```python
from build123d import *

# Parameters (mm, degrees)
SKETCH1_W           = 4.5
SKETCH1_H           = 76
SKETCH2_W           = 19
SKETCH2_H           = 19
BOSS_EXTRUDE1_DEPTH = 6
CHAMFER2_SIZE       = 1
CHAMFER2_SIZE2      = 1.732050808


with BuildPart() as part:
    # Sketch1 → Revolve1 (revolve)
    with BuildSketch(Plane.XY, mode=Mode.PRIVATE) as revolve1_sk:
        with Locations((2.25, 38)):
            Rectangle(SKETCH1_W, SKETCH1_H)
    revolve(revolve1_sk.sketch.rotate(Axis((0, 0, 0), (0, 1, 0)), 90), axis=Axis((0, 0, 0), (0, 1, 0)))  # turned: the seam where the file's is

    # Sketch2 → Boss-Extrude1 (add)
    with BuildSketch(Plane(origin=(0, 0, 0), x_dir=(1, 0, 0), z_dir=(0, 1, 0))):
        Rectangle(SKETCH2_W, SKETCH2_H)
    extrude(amount=-BOSS_EXTRUDE1_DEPTH)

    # Chamfer2
    chamfer2_edges = [part.edges().sort_by_distance(p)[0] for p in [
        (0, 76, 4.5),
    ]]
    chamfer2_side = [part.faces().sort_by_distance(p)[0] for p in [
        (0, 76, 0),
    ]]
    chamfer(chamfer2_edges, length=CHAMFER2_SIZE, length2=CHAMFER2_SIZE2, reference=chamfer2_side[0])


solid = part.part
```
Input: part model. Units: mm. Frame: model coordinates. A direction names the side the tool comes from. Coordinates: 2 decimals unless noted, no trailing zeros. Write each loop counter-clockwise with the first axis right and the second up, starting at its lowest first coordinate (ties: lowest second). Pieces come first, ordered by that corner, then holes. Notation, with made-up numbers: (15.25, 89) - (54.25, 89) arc R20 ccw to (54.25, 105) - close; hole circle Ø1 at (56, -24.5). An arc over 180 degrees is marked (long way). Put each result on its own line as item: value. Start each with the question number.
1) Contact query for flat-ended pins moving along their axis: pin 1 (10 mm diameter, centred on y = 9, z = -2, fed in from -X); pin 2 (3 mm diameter, centred on x = 0.5, y = 53.5, fed in from +Z); pin 3 (8 mm diameter, centred on x = -3, y = 51.5, fed in from -Z). Output: stop coordinate, or through.
2) Cut plane B-B (z = 7.75). Return the cut outline in (x, y).
3) Cut plane A-A (x = 0). Return the cut outline in (y, z).
4) Cut plane D-D (x = -7.5). Return the cut outline in (y, z).
5) Reachability of faces 1 (the face through (-4.4, 0, -2.2)), 2 (the face through (0, -3, 9.5)) from +Z, -Z, +X, -X, +Y, -Y: full face, straight path, thin tool, end or side. Return the list, or none.
6) Ray query, L1, parallel to Y at x = 7.5, z = 2; L2, parallel to Y at x = 3.5, z = -0.25; L3, parallel to Z at x = -1.5, y = 43. Return the intervals inside material, ascending.
7) Cut plane C-C (y = 3). Return the cut outline in (x, z).
Resolved:
1. pin 1: stops at x = -4.5
1. pin 2: stops at z = 4.5
1. pin 3: stops at z = -4.5
2. outline: (-9.5, -6) - (9.5, -6) - (9.5, 0) - (-9.5, 0) - close
3. outline: (-6, -9.5) - (0, -9.5) - (0, -4.5) - (74.27, -4.5) - (76, -3.5) - (76, 3.5) - (74.27, 4.5) - (0, 4.5) - (0, 9.5) - (-6, 9.5) - close
4. outline: (-6, -9.5) - (0, -9.5) - (0, 9.5) - (-6, 9.5) - close
5. face 1: +Y
5. face 2: +Z, +X, -X, +Y, -Y
6. L1: y = -6 to 0
6. L2: y = -6 to 75.98
6. L3: z = -4.24 to 4.24
7. outline: circle Ø9 at (0, 0)
